Study the drawing (mm; zero at the part's minimum x, y, z) and answer. A direction names the side the tool comes from. Round coordinates to 2 decimals unless told otherwise and drop trailing zeros. Order: outer loops, then holes, each group sorted by start corner. A loop starts at its lowest first (then second) coordinate and runs counter-clockwise, first axis right, second up. Notation, with made-up numbers: M -21,39 L 12,39 A19 ccw 12,69 Z; hole C 18.25,59 d3. An arc over 180 degrees is marked long. Put each result on its own line as item: value. Start each with the question number.
1. Consider line 1 (Y direction, x = 74, z = 9.75); line 2 (X direction, y = 28, z = 3); line 3 (Y direction, x = 95.5, z = 0.5). Determine where each line is inside the solid, lowest interval first.
2. Each of these flat-tipped pins is pushed along its axis until it touches: pin 1 Ø7 at (x, z) = (110, 1.5) entering from +Y; pin 2 Ø1.5 at (y, z) = (43, 8.5) entering from +X; pin 3 Ø0.5 at (x, y) = (80, 53.5) entering from +Z; pin 4 Ø7 at (x, z) = (51, 8.5) entering from -Y. Where does it stop, or does it pass through?
3. The part is cut by section C-C (y = 34.5). Give the vertices of the cut face in (x, z).
4. The part is cut by section B-B (x = 90). Give the vertices of the cut face in (y, z), then the cut area to 3 significant figures.
5. The part is cut by section A-A (z = 9.5). Give the vertices of the cut face in (x, y).
6. Which of the six approach directions +Z, -Z, +X, -X, +Y, -Y give full straight-line access (tool end or side, diameter ignored) to the marked faces 3 and 4?
7. The mould has two halves that part along Y. Classify the marked faces 1 and 2: +Y half, -Y half, draft (parallel to the pull), parting line (faces both ways), or undercut.
8. The part is cut by section D-D (y = 16.5). Give the vertices of the cut face in (x, z), then the cut area to 3 significant figures.
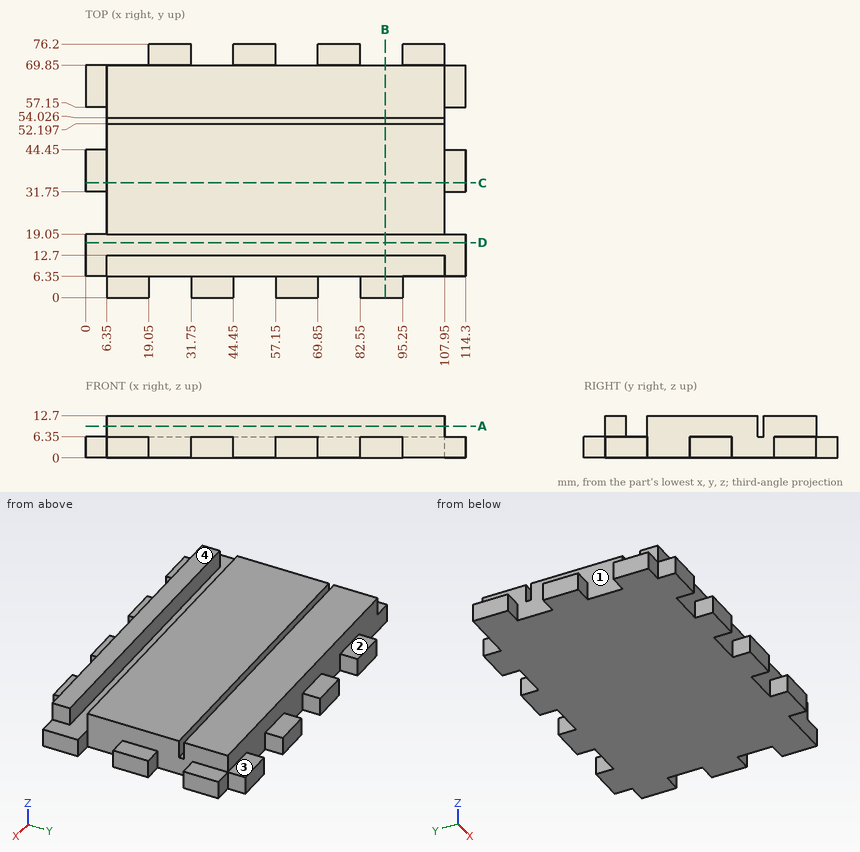
Resolved:
1. line 1: 6.35 to 12.7, 19.05 to 52.2, 54.03 to 69.85
1. line 2: 6.35 to 107.95
1. line 3: 6.35 to 76.2
2. pin 1: y = 76.2
2. pin 2: x = 107.95
2. pin 3: z = 6.35
2. pin 4: y = 6.35
3. outline: M 0,0 L 114.3,0 L 114.3,6.35 L 107.95,6.35 L 107.95,12.7 L 6.35,12.7 L 6.35,6.35 L 0,6.35 Z
4. outline: M 0,0 L 69.85,0 L 69.85,12.7 L 54.03,12.7 L 54.03,6.35 L 52.2,6.35 L 52.2,12.7 L 19.05,12.7 L 19.05,6.35 L 12.7,6.35 L 12.7,12.7 L 6.35,12.7 L 6.35,6.35 L 0,6.35 Z
4. area: 795 mm2
5. outline: M 6.35,6.35 L 107.95,6.35 L 107.95,12.7 L 6.35,12.7 Z; M 6.35,19.05 L 107.95,19.05 L 107.95,52.2 L 6.35,52.2 Z; M 6.35,54.03 L 107.95,54.03 L 107.95,69.85 L 6.35,69.85 Z
6. face 3: +Z, +X, -X, +Y
6. face 4: +Z, +X, -X, +Y, -Y
7. face 1: undercut
7. face 2: draft
8. outline: M 0,0 L 114.3,0 L 114.3,6.35 L 0,6.35 Z
8. area: 726 mm2
